```python
from build123d import *

# Parameters (mm, degrees)
ESBO_O1_W                = 150
ESBO_O1_H                = 80
RESSALTO_EXTRUS_O1_DEPTH = 20
ESBO_O2_W                = 140
ESBO_O2_H                = 10
CORTE_EXTRUS_O1_DEPTH    = 172.172427686
ESBO_O3_W                = 10
ESBO_O3_H                = 70
CORTE_EXTRUS_O2_DEPTH    = 172.172427686
ESBO_O4_W                = 45
ESBO_O4_H                = 70
ESBO_O4_W_2              = 90
CORTE_EXTRUS_O3_DEPTH    = 15
ESBO_O5_W                = 5.002119461
ESBO_O5_H                = 20
RESSALTO_EXTRUS_O2_DEPTH = 80
ESBO_O6_W                = 20
ESBO_O6_H                = 10
RESSALTO_EXTRUS_O3_DEPTH = 5
ESBO_O7_W                = 20
ESBO_O7_H                = 10
RESSALTO_EXTRUS_O4_DEPTH = 5


with BuildPart() as part:
    # Esboço1 → Ressalto-extrusão1 (new body)
    with BuildSketch(Plane.XY):
        with Locations((75, 40)):
            Rectangle(ESBO_O1_W, ESBO_O1_H)
    extrude(amount=RESSALTO_EXTRUS_O1_DEPTH)

    # Esboço2 → Corte-extrusão1 (cut, through all)
    with BuildSketch(Plane(origin=(0, 80, 0), x_dir=(1, 0, 0), z_dir=(0, 1, 0))):
        with Locations((75, -10)):
            Rectangle(ESBO_O2_W, ESBO_O2_H)
    extrude(amount=-CORTE_EXTRUS_O1_DEPTH, mode=Mode.SUBTRACT)

    # Esboço3 → Corte-extrusão2 (cut, through all)
    with BuildSketch(Plane.ZY):
        with Locations((10, 40)):
            Rectangle(ESBO_O3_W, ESBO_O3_H)
    extrude(amount=-CORTE_EXTRUS_O2_DEPTH, mode=Mode.SUBTRACT)

    # Esboço4 → Corte-extrusão3 (cut)
    with BuildSketch(Plane.XY.offset(20)):
        with Locations((27.5, 40)):
            Rectangle(ESBO_O4_W, ESBO_O4_H)
        with Locations((100, 40)):
            Rectangle(ESBO_O4_W_2, ESBO_O4_H)
    extrude(amount=-CORTE_EXTRUS_O3_DEPTH, mode=Mode.SUBTRACT)

    # Esboço5 → Ressalto-extrusão2 (add)
    with BuildSketch(Plane(origin=(0, 80, 0), x_dir=(1, 0, 0), z_dir=(0, 1, 0))):
        with Locations((52.501059731, -10)):
            Rectangle(ESBO_O5_W, ESBO_O5_H)
    extrude(amount=-RESSALTO_EXTRUS_O2_DEPTH)

    # Esboço6 → Ressalto-extrusão3 (add)
    with BuildSketch(Plane.ZY):
        with Locations((10, 40)):
            Rectangle(ESBO_O6_W, ESBO_O6_H)
    extrude(amount=-RESSALTO_EXTRUS_O3_DEPTH)

    # Esboço7 → Ressalto-extrusão4 (add)
    with BuildSketch(Plane(origin=(150, 0, 0), x_dir=(0, 0, -1), z_dir=(1, 0, 0))):
        with Locations((-10, 40)):
            Rectangle(ESBO_O7_W, ESBO_O7_H)
    extrude(amount=-RESSALTO_EXTRUS_O4_DEPTH)


solid = part.part
```
Part model, mm, in its own coordinate system. A direction names the side the tool comes from. Round coordinates to 2 decimals unless told otherwise and drop trailing zeros. Order: outer loops, then holes, each group sorted by start corner. A loop starts at its lowest first (then second) coordinate and runs counter-clockwise, first axis right, second up. Notation, with made-up numbers: M 76,80.25 L 106,80.25 A18 cw 106,91.25 Z; hole C 22.25,5 d7. An arc over 180 degrees is marked long. Answer in a Markdown table with one row per item. Add a question column.
Q1. Mould opens along Y. For faces 5 (the face through (147, 75, 10)), 6 (the face through (5, 78, 10)), 7 (the face through (74, 80, 3)) say: +Y half, -Y half, draft (parallel to the pull), parting line (faces both ways), or undercut.
Q2. Cut at D-D on z = 18. Give the cut face in (x, y), and give its area (3 significant figures).
Q3. Wall check: L1, parallel to X at y = 40, z = 9.25; L2, parallel to Z at x = 31, y = 70; L3, parallel to X at y = 13, z = 6.25. Give the ranges that are in metal, low to high. Write a range as from..to.
Q4. Cut at B-B on y = 33.5. Give the cut face in (x, z), and give its area (3 significant figures).
Q5. 3-axis set-ups, long thin cutter, end or side, ignore diameter. For faces 1 (the face through (145, 3, 10)), 2 (the face through (99, 75, 18)), 3 (the face through (2, 60, 15)), 4 (the face through (0, 39, 10)): which of +Z, -Z, +X, -X, +Y, -Y reach the whole face in a straight line?
Q6. Cut at C-C on x = 28. Give the cut face in (y, z), and give its area (3 significant figures).
Q7. Cut at A-A on z = 7.5. Give the cut face in (x, y), and give its area (3 significant figures).
Q8. Pin check, flat tips, straight feed: pin 1 (12 mm diameter, centred on x = 36, y = 65.5, fed in from +Z); pin 2 (6 mm diameter, centred on x = 108.5, z = 7.5, fed in from +Y); pin 3 (1.5 mm diameter, centred on x = 28, z = 13, fed in from -Y). Stop position of each tip, or through.
Established:
| question | item | result |
|---|---|---|
| 1 | face 5 | undercut |
| 1 | face 6 | draft |
| 1 | face 7 | +Y half |
| 2 | outline | M 0,0 L 150,0 L 150,80 L 0,80 Z; hole M 5,5 L 50,5 L 50,75 L 5,75 Z; hole M 55,5 L 145,5 L 145,75 L 55,75 Z |
| 2 | area | 2,550 mm2 |
| 3 | L1 | x = 0..5, 50..55, 145..150 |
| 3 | L2 | z = 0..5 |
| 3 | L3 | x = 50..55 |
| 4 | outline | M 0,0 L 150,0 L 150,5 L 55,5 L 55,20 L 50,20 L 50,5 L 0,5 Z; M 0,15 L 5,15 L 5,20 L 0,20 Z; M 145,15 L 150,15 L 150,20 L 145,20 Z |
| 4 | area | 875 mm2 |
| 5 | face 1 | +Y, -Y |
| 5 | face 2 | +Z |
| 5 | face 3 | -X |
| 5 | face 4 | +Z, -Z, -X, +Y, -Y |
| 6 | outline | M 0,0 L 80,0 L 80,5 L 0,5 Z; M 0,15 L 5,15 L 5,20 L 0,20 Z; M 75,15 L 80,15 L 80,20 L 75,20 Z |
| 6 | area | 450 mm2 |
| 7 | outline | M 0,0 L 5,0 L 5,5 L 0,5 Z; M 0,35 L 5,35 L 5,45 L 0,45 Z; M 0,75 L 5,75 L 5,80 L 0,80 Z; M 50,0 L 55,0 L 55,80 L 50,80 Z; M 145,0 L 150,0 L 150,5 L 145,5 Z; M 145,35 L 150,35 L 150,45 L 145,45 Z; M 145,75 L 150,75 L 150,80 L 145,80 Z |
| 7 | area | 600 mm2 |
| 8 | pin 1 | stops at z = 5 |
| 8 | pin 2 | stops at y = 80 |
| 8 | pin 3 | passes through |
